```python
from build123d import *

# Parameters (mm, degrees)
SKETCH_1_R          = 1.45
EXTRUDE_1_DEPTH     = 3
EXTRUDE_2_DEPTH     = 3
SKETCH_4_W          = 43.75
SKETCH_4_H          = 58.75
CUT_EXTRUDE_2_DEPTH = 79.02002948
SKETCH_5_W          = 15
SKETCH_5_H          = 15
CUT_EXTRUDE_3_DEPTH = 79.02002948
SKETCH_6_W          = 15
SKETCH_6_H          = 3
CUT_EXTRUDE_4_DEPTH = 0.1
FILLET_1_R          = 3


with BuildPart() as part:
    # 草图1 → 凸台-拉伸1 (new body)
    with BuildSketch(Plane(origin=(0, 0, 0), x_dir=(1, 0, 0), z_dir=(0, 1, 0))):
        Polygon((-51.25, 0), (0, 0), (51.25, 0), (51.25, -15), (7.5, -15), (7.5, -58.75), (-7.5, -58.75), (-7.5, -15), (-51.25, -15), align=None)
        with Locations(Location((0, -7.5, 0), (0, 0, 270))):
            Circle(SKETCH_1_R, mode=Mode.SUBTRACT)
        with Locations(Location((0, -33.75, 0), (0, 0, 270))):
            Circle(SKETCH_1_R, mode=Mode.SUBTRACT)
        with Locations(Location((0, -53.75, 0), (0, 0, 270))):
            Circle(SKETCH_1_R, mode=Mode.SUBTRACT)
        with Locations(Location((-26.25, -7.5, 0), (0, 0, 270))):
            Circle(SKETCH_1_R, mode=Mode.SUBTRACT)
        with Locations(Location((-46.25, -7.5, 0), (0, 0, 270))):
            Circle(SKETCH_1_R, mode=Mode.SUBTRACT)
        with Locations(Location((46.25, -7.5, 0), (0, 0, 90))):
            Circle(SKETCH_1_R, mode=Mode.SUBTRACT)
        with Locations(Location((26.25, -7.5, 0), (0, 0, 90))):
            Circle(SKETCH_1_R, mode=Mode.SUBTRACT)
    extrude(amount=EXTRUDE_1_DEPTH)

    # 草图2 → 凸台-拉伸2 (add)
    with BuildSketch(Plane(origin=(0, 3, 0), x_dir=(1, 0, 0), z_dir=(0, 1, 0))):
        Polygon((-51.25, -15), (-7.5, -58.75), (-7.5, -44.607864376), (-37.107864376, -15), align=None)
        Polygon((37.107864376, -15), (51.25, -15), (7.5, -58.75), (7.5, -44.607864376), align=None)
    extrude(amount=-EXTRUDE_2_DEPTH)

    # 草图4 → 切除-拉伸2 (cut, through all)
    with BuildSketch(Plane(origin=(0, 3, 0), x_dir=(1, 0, 0), z_dir=(0, 1, 0))):
        with Locations((29.375, -29.375)):
            Rectangle(SKETCH_4_W, SKETCH_4_H)
    extrude(amount=-CUT_EXTRUDE_2_DEPTH, mode=Mode.SUBTRACT)

    # 草图5 → 切除-拉伸3 (cut, through all)
    with BuildSketch(Plane(origin=(0, 3, 0), x_dir=(1, 0, 0), z_dir=(0, 1, 0))):
        with Locations((0, -22.5)):
            Rectangle(SKETCH_5_W, SKETCH_5_H)
    extrude(amount=-CUT_EXTRUDE_3_DEPTH, mode=Mode.SUBTRACT)

    # 草图6 → 切除-拉伸4 (cut)
    with BuildSketch(Plane(origin=(0, 0, 30), x_dir=(-1, 0, 0), z_dir=(0, 0, -1))):
        with Locations((0, 1.5)):
            Rectangle(SKETCH_6_W, SKETCH_6_H)
    extrude(amount=-CUT_EXTRUDE_4_DEPTH, mode=Mode.SUBTRACT)

    # 圆角1
    fillet_1_edges = [part.edges().sort_by_distance(p)[0] for p in [
        (7.5, 1.5, 15),
        (-7.5, 1.5, 30.1),
        (7.5, 1.5, 30.1),
        (-51.25, 1.5, 0),
        (7.5, 1.5, 58.75),
        (-7.5, 1.5, 58.75),
        (-51.25, 1.5, 15),
        (-7.5, 1.5, 44.607864376),
        (-37.107864376, 1.5, 15),
        (7.5, 1.5, 0),
    ]]
    fillet(fillet_1_edges, radius=FILLET_1_R)


solid = part.part
```
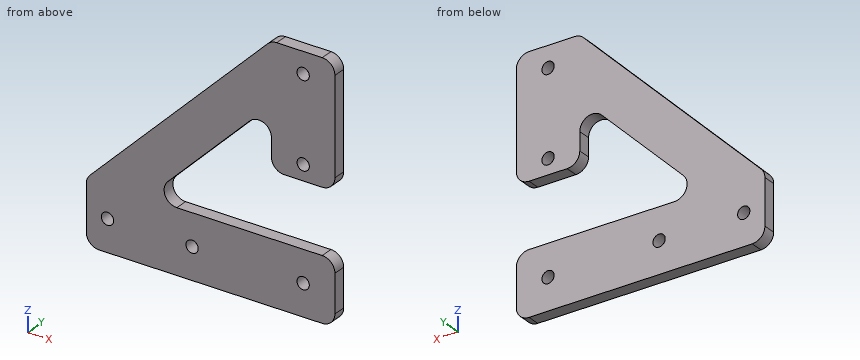
Geometry: final body of the model. Coordinates: model frame, mm. Round coordinates to 2 decimals unless told otherwise and drop trailing zeros. Order: outer loops, then holes, each group sorted by start corner. A loop starts at its lowest first (then second) coordinate and runs counter-clockwise, first axis right, second up. Notation, with made-up numbers: (-25.75, -38) - (-19.75, -38) arc R9 ccw to (-19.75, -26) - close; hole circle Ø8 at (59, 15). An arc over 180 degrees is marked (long way). Use CSV: the item, a comma, the result in double quotes. Start each with the question number.
Q1. Section query A-A (z = 7.5). Return loops of the section in (x, y), and give its area (3 significant figures).
Q2. First-contact query: pin 1 (2.5 mm diameter, centred on x = 0, z = 7.5, fed in from -Y); pin 2 (1.5 mm diameter, centred on y = 1, z = 35, fed in from -X). Flat tips, straight axial feed; report the tip coordinate or a pass-through.
Q3. Section query B-B (x = -46.25). Return loops of the section in (y, z).
Q4. Section query D-D (x = 0). Return loops of the section in (y, z).
Q5. Section query C-C (y = 1.15). Return loops of the section in (x, z).
Q6. Material intervals for line 1 along X through (y, z) = (2.1, 7.5); line 2 along X through (y, z) = (0.65, 33.75); line 3 along Z through (x, y) = (-25.5, 2.3), sorted ascending. Write a range as from..to.
Result set:
1,outline,"(-51.25, 0) - (-47.7, 0) - (-47.7, 3) - (-51.25, 3) - close; (-44.8, 0) - (-27.7, 0) - (-27.7, 3) - (-44.8, 3) - close; (-24.8, 0) - (-1.45, 0) - (-1.45, 3) - (-24.8, 3) - close; (1.45, 0) - (7.5, 0) - (7.5, 3) - (1.45, 3) - close"
1,area,"150 mm2"
2,pin 1,"passes through"
2,pin 2,"stops at x = -32"
3,outline,"(0, 0) - (3, 0) - (3, 6.05) - (0, 6.05) - close; (0, 8.95) - (3, 8.95) - (3, 20) - (0, 20) - close"
4,outline,"(0, 0) - (3, 0) - (3, 6.05) - (0, 6.05) - close; (0, 8.95) - (3, 8.95) - (3, 15) - (0, 15) - close; (0, 30.1) - (3, 30.1) - (3, 32.3) - (0, 32.3) - close; (0, 35.2) - (3, 35.2) - (3, 52.3) - (0, 52.3) - close; (0, 55.2) - (3, 55.2) - (3, 58.75) - (0, 58.75) - close"
5,outline,"(-51.25, 3) arc R3 ccw to (-48.25, 0) - (4.5, 0) arc R3 ccw to (7.5, 3) - (7.5, 12) arc R3 ccw to (4.5, 15) - (-29.87, 15) arc R3 cw to (-31.99, 20.12) - (-12.62, 39.49) arc R3 cw to (-7.5, 37.37) - (-7.5, 33.1) arc R3 ccw to (-4.5, 30.1) - (4.5, 30.1) arc R3 ccw to (7.5, 33.1) - (7.5, 55.75) arc R3 ccw to (4.5, 58.75) - (-6.26, 58.75) arc R3 ccw to (-8.38, 57.87) - (-50.37, 15.88) arc R3 ccw to (-51.25, 13.76) - close; hole circle Ø2.9 at (-46.25, 7.5); hole circle Ø2.9 at (-26.25, 7.5); hole circle Ø2.9 at (0, 7.5); hole circle Ø2.9 at (0, 33.75); hole circle Ø2.9 at (0, 53.75)"
6,line 1,"x = -51.25..-47.7, -44.8..-27.7, -24.8..-1.45, 1.45..7.5"
6,line 2,"x = -32.5..-18.36, -7.5..-1.45, 1.45..7.5"
6,line 3,"z = 0..6.26, 8.74..15, 26.61..40.75"
